Verification items for the finished model (mm, model axes). Face numbers are marked on the shaded views. A direction names the side the tool comes from. Round coordinates to 2 decimals unless told otherwise and drop trailing zeros. Write each loop counter-clockwise with the first axis right and the second up, starting at its lowest first coordinate (ties: lowest second). Pieces come first, ordered by that corner, then holes. Notation, with made-up numbers: (86.25, 62) - (94.25, 62) arc R25 cw to (94.25, 96) - close; hole circle Ø7 at (47, -18.5). An arc over 180 degrees is marked (long way). Answer as a JSON object with one key per item and string values.
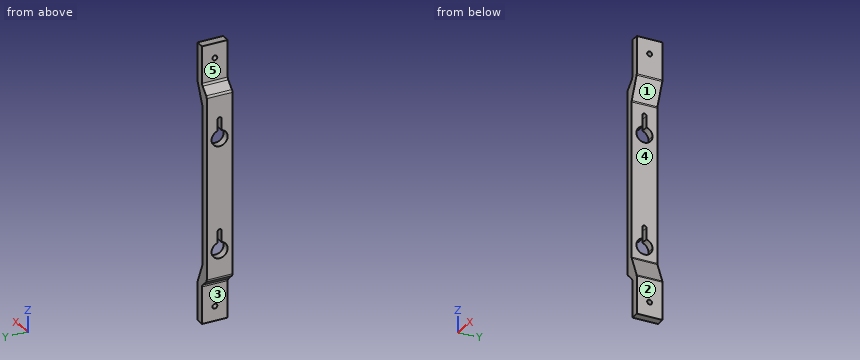
```python
from build123d import *

# Parameters (mm, degrees)
F1_DEPTH = 40
F2_R     = 5
F3_R     = 5
F5_D     = 7.5
F7_DEPTH = 12


with BuildPart() as f1:
    # F0 (on Front) → F1 (new body)
    with BuildSketch(Plane.XZ):
        Polygon((8.02879, 156.936201), (-6, 144), (6, 144), (21.253023, 156.936201), (21.253023, 216.936201), (8.02879, 216.936201), align=None)
        Polygon((6, 144), (-6, 144), (-6, -144), (6, -144), (6, -122.299686), (6, 122.299686), align=None)
        Polygon((21.253023, 156.936201), (6, 144), (6, 122.299686), align=None)
        Polygon((6, -144), (-6, -144), (8.02879, -156.936201), (8.02879, -216.936201), (21.253023, -216.936201), (21.253023, -156.936201), align=None)
        Polygon((6, -122.299686), (6, -144), (21.253023, -156.936201), align=None)
    extrude(amount=F1_DEPTH)

    # F2
    f2_edges = [f1.edges().sort_by_distance(p)[0] for p in [
        (6, -20, -122.299686),
        (21.253023, -20, -156.936201),
        (8.02879, -20, -156.936201),
        (-6, -20, -144),
        (-6, -20, 144),
        (6, -20, 122.299686),
        (21.253023, -20, 156.936201),
    ]]
    fillet(f2_edges, radius=F2_R)

    # F3
    f3_edges = [f1.edges().sort_by_distance(p)[0] for p in [
        (8.02879, -20, 156.936201),
    ]]
    fillet(f3_edges, radius=F3_R)

    # F5 (through all)
    with Locations(Plane.YZ.offset(21.253023)):
        with Locations((-20, 194), (-20, -194)):
            Hole(F5_D / 2)

    # F6 (on face) → F7 (cut)
    with BuildSketch(Plane.YZ.offset(6)):
        with BuildLine():
            Line((-17, -100), (-17, -87.865339))
            ThreePointArc((-17, -87.865339), (-18.488918, -87.591671), (-20, -87.5))
            ThreePointArc((-20, -87.5), (-21.511082, -87.591671), (-23, -87.865339))
            Line((-23, -87.865339), (-23, -100))
            ThreePointArc((-23, -100), (-20, -103), (-17, -100))
        make_face()
        with BuildLine():
            ThreePointArc((-23, -87.865339), (-27.705518, -109.84251), (-7.5, -100))
            ThreePointArc((-7.5, -100), (-10.15749, -92.294482), (-17, -87.865339))
            Line((-17, -87.865339), (-17, -100))
            ThreePointArc((-17, -100), (-20, -103), (-23, -100))
            Line((-23, -100), (-23, -87.865339))
        make_face()
        with BuildLine():
            ThreePointArc((-23, 87.134661), (-27.705518, 65.15749), (-7.5, 75))
            ThreePointArc((-7.5, 75), (-10.15749, 82.705518), (-17, 87.134661))
            Line((-17, 87.134661), (-17, 75))
            ThreePointArc((-17, 75), (-20, 72), (-23, 75))
            Line((-23, 75), (-23, 87.134661))
        make_face()
        with BuildLine():
            Line((-17, 75), (-17, 87.134661))
            ThreePointArc((-17, 87.134661), (-18.488918, 87.408329), (-20, 87.5))
            ThreePointArc((-20, 87.5), (-21.511082, 87.408329), (-23, 87.134661))
            Line((-23, 87.134661), (-23, 75))
            ThreePointArc((-23, 75), (-20, 72), (-17, 75))
        make_face()
        with BuildLine():
            ThreePointArc((-20, 87.5), (-18.488918, 87.408329), (-17, 87.134661))
            Line((-17, 87.134661), (-17, 105))
            ThreePointArc((-17, 105), (-20, 108), (-23, 105))
            Line((-23, 105), (-23, 87.134661))
            ThreePointArc((-23, 87.134661), (-21.511082, 87.408329), (-20, 87.5))
        make_face()
        with BuildLine():
            ThreePointArc((-20, -87.5), (-18.488918, -87.591671), (-17, -87.865339))
            Line((-17, -87.865339), (-17, -70))
            ThreePointArc((-17, -70), (-20, -67), (-23, -70))
            Line((-23, -70), (-23, -87.865339))
            ThreePointArc((-23, -87.865339), (-21.511082, -87.591671), (-20, -87.5))
        make_face()
    extrude(amount=-F7_DEPTH, mode=Mode.SUBTRACT)


solid = f1.part
```
Q1. Material ranges on line 1 along Y through (x, z) = (-0.75, -100); line 2 along Y through (x, z) = (12.5, 194); line 3 along Z through (x, y) = (3.75, -28.5), recorded low to high. Write a range as [from, to].
Geometry check:
{"line 1": "y = [-40, -32.5], [-7.5, 0]", "line 2": "y = [-40, -23.75], [-16.25, 0]", "line 3": "z = [-152.99, -109.17], [-90.83, 65.83], [84.17, 152.99]"}
Q2. Section check A-A, the plane z = -107.5. Record the cut outline in (x, y), then the cut area to 3 significant figures.
Geometry check:
{"outline": "(-6, -40) - (6, -40) - (6, -30) - (-6, -30) - close; (-6, -10) - (6, -10) - (6, 0) - (-6, 0) - close", "area": "240 mm2"}
Q3. Release check for a two-part mould opening along Z. For the marked faces 4 and 5 record: released by +Z, released by -Z, zero draft, split by the parting line, or undercut.
Geometry check:
{"face 4": "undercut", "face 5": "zero draft"}
Q4. Section check C-C, the plane y = -4. Record the cut outline in (x, z), then the cut area to 3 significant figures.
Geometry check:
{"outline": "(-6, -141.81) arc R5 ccw to (-4.39, -145.49) - (6.42, -155.45) arc R5 cw to (8.03, -159.13) - (8.03, -216.94) - (21.25, -216.94) - (21.25, -157.99) arc R5 ccw to (20.83, -155.97) - (6.42, -123.26) arc R5 cw to (6, -121.25) - (6, 121.25) arc R5 cw to (6.42, 123.26) - (20.83, 155.97) arc R5 ccw to (21.25, 157.99) - (21.25, 216.94) - (8.03, 216.94) - (8.03, 159.13) arc R5 cw to (6.42, 155.45) - (-4.39, 145.49) arc R5 ccw to (-6, 141.81) - close", "area": "5,700 mm2"}
Q5. Section check D-D, the plane z = 81.5. Record the cut outline in (x, y), then the cut area to 3 significant figures.
Geometry check:
{"outline": "(-6, -40) - (6, -40) - (6, -30.68) - (-6, -30.68) - close; (-6, -9.32) - (6, -9.32) - (6, 0) - (-6, 0) - close", "area": "224 mm2"}
Q6. Section check B-B, the plane x = 17. Record the cut outline in (y, z).
Geometry check:
{"outline": "(-40, -216.94) - (0, -216.94) - (0, -147.28) - (-40, -147.28) - close; (-40, 147.28) - (0, 147.28) - (0, 216.94) - (-40, 216.94) - close; hole circle Ø7.5 at (-20, -194); hole circle Ø7.5 at (-20, 194)"}
Q7. Set-up check for the marked faces 1, 2 and 3: record each of +Z, -Z, +X, -X, +Y, -Y from which the full face is reachable in a straight line by a thin tool's end or side.
Geometry check:
{"face 1": "+X, +Y, -Y", "face 2": "+Z, -Z, +X, +Y, -Y", "face 3": "-Z, -X, +Y, -Y"}
Q8. Gauge pin test, flat ends, axial feed: P1, Ø3, axis at y = -5.5, z = -111, coming from the +X side; P2, Ø3, axis at x = 5.5, y = -11, coming from the +Z side; P3, Ø4, axis at y = -15.5, z = -150, coming from the -X side. Record the tip position at first contact, or that the pin passes through.
Geometry check:
{"P1": "stops at x = 6", "P2": "stops at z = 156.09", "P3": "stops at x = -1.66"}
